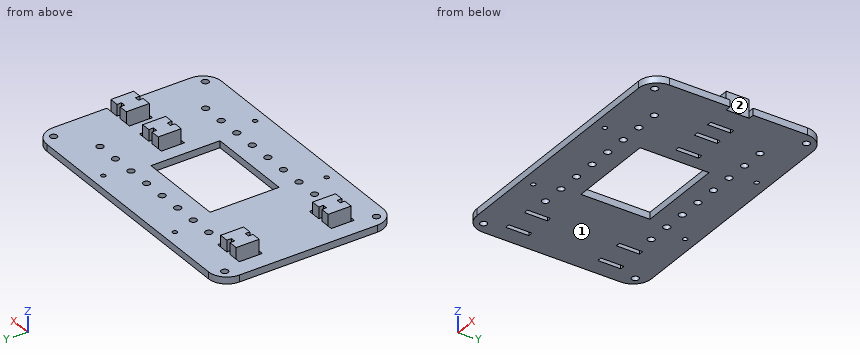
from build123d import *

# Parameters (mm, degrees)
SKETCH_2_W          = 120
SKETCH_2_H          = 76
SKETCH_2_R          = 1
EXTRUDE_2_DEPTH     = 3
SKETCH_3_W          = 38
SKETCH_3_H          = 30
CUT_EXTRUDE_1_DEPTH = 3
EXTRUDE_3_DEPTH     = 5
SKETCH_7_W          = 2
SKETCH_7_H          = 10
SKETCH_7_W_2        = 3
CUT_EXTRUDE_2_DEPTH = 5
SKETCH_9_R          = 1.5
CUT_EXTRUDE_3_DEPTH = 5
FILLET_1_R          = 8
SKETCH_10_R         = 1.5
CUT_EXTRUDE_4_DEPTH = 5


with BuildPart() as part:
    # 草图2 → 凸台-拉伸2 (new body)
    with BuildSketch(Plane.XY):
        Rectangle(SKETCH_2_W, SKETCH_2_H)
        with Locations((-23, 33)):
            Circle(SKETCH_2_R, mode=Mode.SUBTRACT)
        with Locations(Location((23, 33, 0), (0, 0, 180))):
            Circle(SKETCH_2_R, mode=Mode.SUBTRACT)
        with Locations((23, -33)):
            Circle(SKETCH_2_R, mode=Mode.SUBTRACT)
        with Locations(Location((-23, -33, 0), (0, 0, 180))):
            Circle(SKETCH_2_R, mode=Mode.SUBTRACT)
    extrude(amount=EXTRUDE_2_DEPTH)

    # 草图3 → 切除-拉伸1 (cut)
    with BuildSketch(Plane.XY.offset(3)):
        Rectangle(SKETCH_3_W, SKETCH_3_H)
    extrude(amount=-CUT_EXTRUDE_1_DEPTH, mode=Mode.SUBTRACT)

    # 草图6 → 凸台-拉伸3 (add)
    with BuildSketch(Plane.XY.offset(3)):
        Polygon((-50.570869285, 25), (-50.570869285, 15), (-46.570869285, 15), (-46.570869285, 17), (-44.570869285, 17), (-44.570869285, 15), (-40.570869285, 15), (-40.570869285, 25), (-44.570869285, 25), (-44.570869285, 23), (-46.570869285, 23), (-46.570869285, 25), align=None)
        Polygon((-50.570869285, -15), (-50.570869285, -25), (-46.570869285, -25), (-46.570869285, -23), (-44.570869285, -23), (-44.570869285, -25), (-40.570869285, -25), (-40.570869285, -15), (-44.570869285, -15), (-44.570869285, -17), (-46.570869285, -17), (-46.570869285, -15), align=None)
        Polygon((31, -1.582947544), (33, -1.582947544), (33, -3.582947544), (37, -3.582947544), (37, 6.417052456), (33, 6.417052456), (33, 4.417052456), (31, 4.417052456), (31, 6.417052456), (27, 6.417052456), (27, -3.582947544), (31, -3.582947544), align=None)
        Polygon((53.519832093, 6.417052456), (53.519832093, 4.417052456), (51.519832093, 4.417052456), (51.519832093, 6.417052456), (47.519832093, 6.417052456), (47.519832093, -3.582947544), (51.519832093, -3.582947544), (51.519832093, -1.582947544), (53.519832093, -1.582947544), (53.519832093, -3.582947544), (57.519832093, -3.582947544), (57.519832093, 6.417052456), align=None)
    extrude(amount=EXTRUDE_3_DEPTH)

    # 草图7 → 切除-拉伸2 (cut)
    with BuildSketch(Plane.XY.offset(3)):
        with Locations((-51.570869285, 20)):
            Rectangle(SKETCH_7_W, SKETCH_7_H)
        with Locations((-39.570869285, 20)):
            Rectangle(SKETCH_7_W, SKETCH_7_H)
        with Locations((-51.570869285, -20)):
            Rectangle(SKETCH_7_W, SKETCH_7_H)
        with Locations((-39.570869285, -20)):
            Rectangle(SKETCH_7_W, SKETCH_7_H)
        with Locations((26, 1.417052456)):
            Rectangle(SKETCH_7_W, SKETCH_7_H)
        with Locations((38, 1.417052456)):
            Rectangle(SKETCH_7_W, SKETCH_7_H)
        with Locations((46.519832093, 1.417052456)):
            Rectangle(SKETCH_7_W, SKETCH_7_H)
        with Locations((59.019832093, 1.417052456)):
            Rectangle(SKETCH_7_W_2, SKETCH_7_H)
    extrude(amount=-CUT_EXTRUDE_2_DEPTH, mode=Mode.SUBTRACT)

    # 草图9 → 切除-拉伸3 (cut)
    with BuildSketch(Plane.XY.offset(3)):
        with Locations((0, -23)):
            Circle(SKETCH_9_R)
        with Locations((10, -23)):
            Circle(SKETCH_9_R)
        with Locations((20, -23)):
            Circle(SKETCH_9_R)
        with Locations((30, -23)):
            Circle(SKETCH_9_R)
        with Locations((40, -23)):
            Circle(SKETCH_9_R)
        with Locations((-30, -23)):
            Circle(SKETCH_9_R)
        with Locations((-20, -23)):
            Circle(SKETCH_9_R)
        with Locations((-10, -23)):
            Circle(SKETCH_9_R)
        with Locations((-10, 23)):
            Circle(SKETCH_9_R)
        with Locations((-20, 23)):
            Circle(SKETCH_9_R)
        with Locations((-30, 23)):
            Circle(SKETCH_9_R)
        with Locations((40, 23)):
            Circle(SKETCH_9_R)
        with Locations((30, 23)):
            Circle(SKETCH_9_R)
        with Locations((20, 23)):
            Circle(SKETCH_9_R)
        with Locations((10, 23)):
            Circle(SKETCH_9_R)
        with Locations((0, 23)):
            Circle(SKETCH_9_R)
    extrude(amount=-CUT_EXTRUDE_3_DEPTH, mode=Mode.SUBTRACT)

    # 圆角1
    fillet_1_edges = [part.edges().sort_by_distance(p)[0] for p in [
        (60, -38, 1.5),
        (-60, -38, 1.5),
        (-60, 38, 1.5),
        (60, 38, 1.5),
    ]]
    fillet(fillet_1_edges, radius=FILLET_1_R)

    # 草图10 → 切除-拉伸4 (cut)
    with BuildSketch(Plane.XY.offset(3)):
        with Locations((-55, 33)):
            Circle(SKETCH_10_R)
        with Locations((55, 33)):
            Circle(SKETCH_10_R)
        with Locations((55, -33)):
            Circle(SKETCH_10_R)
        with Locations((-55, -33)):
            Circle(SKETCH_10_R)
    extrude(amount=-CUT_EXTRUDE_4_DEPTH, mode=Mode.SUBTRACT)


solid = part.part
Design review of the part built by this model. Coordinates are the model's own, in mm. Face numbers are marked on the shaded views. Coordinates: 2 decimals unless noted, no trailing zeros. Loops run counter-clockwise (first coordinate to the right, second up) from the corner with the lowest first, then second, coordinate; pieces in that order, holes last.
Item 1: Add section D-D (z = 4.75). Give the number of separate pieces and of enclosed holes in the cut face, and give its area (3 significant figures).
Completed:
separate pieces: 4
enclosed holes: 0
area: 368 mm2
Item 2: Add section B-B (x = -10). Write out the cut boundary in (y, z).
Completed:
outline: (-38, 0) - (-24.5, 0) - (-24.5, 3) - (-38, 3) - close; (-21.5, 0) - (-15, 0) - (-15, 3) - (-21.5, 3) - close; (15, 0) - (21.5, 0) - (21.5, 3) - (15, 3) - close; (24.5, 0) - (38, 0) - (38, 3) - (24.5, 3) - close
Item 3: Clearance check with flat-ended pins moving along their axes: pin 1 (2 mm diameter, centred on y = 16.5, z = 6, fed in from -X); pin 2 (1 mm diameter, centred on y = -2.5, z = 5.5, fed in from -X); pin 3 (3 mm diameter, centred on x = 11.5, y = 21.5, fed in from +Z). State where each tip first meets the part, or that it passes through.
Completed:
pin 1: stops at x = -50.57
pin 2: stops at x = 27
pin 3: stops at z = 3
Item 4: Wall thickness on L1, parallel to Y at x = -20, z = 1.25; L2, parallel to Y at x = -47.5, z = 4.75; L3, parallel to Y at x = -55, z = 2.35: over which ranges is each line inside the solid? List them lowest first.
Completed:
L1: y = -38 to -24.5, -21.5 to 21.5, 24.5 to 38
L2: y = -25 to -15, 15 to 25
L3: y = -37.42 to -34.5, -31.5 to 31.5, 34.5 to 37.42
Item 5: Add section C-C (y = -7). Write out the cut boundary in (x, z), and give its area (3 significant figures).
Completed:
outline: (-60, 0) - (-19, 0) - (-19, 3) - (-60, 3) - close; (19, 0) - (60, 0) - (60, 3) - (19, 3) - close
area: 246 mm2
Item 6: Add section A-A (y = 1). Write out the cut boundary in (x, z), and give its area (3 significant figures).
Completed:
outline: (-60, 0) - (-19, 0) - (-19, 3) - (-60, 3) - close; (19, 0) - (25, 0) - (25, 3) - (19, 3) - close; (27, 0) - (37, 0) - (37, 8) - (27, 8) - close; (39, 0) - (45.52, 0) - (45.52, 3) - (39, 3) - close; (47.52, 0) - (57.52, 0) - (57.52, 8) - (47.52, 8) - close
area: 321 mm2
Item 7: Draft analysis for pull direction Y (two halves, no side actions). For the marked faces 1 and 2, state which applies: pulls with the +Y half, pulls with the -Y half, needs draft (parallel to the pull), parting line crosses it, or undercut.
Completed:
face 1: needs draft
face 2: undercut
